```python
from build123d import *

# Parameters (mm, degrees)
CROQUIS1_W              = 50
CROQUIS1_H              = 61
SALIENTE_EXTRUIR1_DEPTH = 3
CROQUIS2_R              = 1.6
CORTAR_EXTRUIR1_DEPTH   = 40.550600501
CROQUIS4_R              = 1
CROQUIS4_W              = 23
CROQUIS4_H              = 13
CORTAR_EXTRUIR3_DEPTH   = 10
CROQUIS7_R              = 1.6
CORTAR_EXTRUIR5_DEPTH   = 10
CROQUIS5_W              = 13
CROQUIS5_H              = 7
CROQUIS5_W_2            = 26
CROQUIS5_H_2            = 11.5
CORTAR_EXTRUIR4_DEPTH   = 10
REDONDEO4_R             = 1.5
SALIENTE_EXTRUIR2_DEPTH = 3
REDONDEO3_DEPTH         = 3
REDONDEO3_2_DEPTH       = 3
REDONDEO5_R             = 2
CROQUIS9_R              = 1.6
CORTAR_EXTRUIR6_DEPTH   = 60.41214848
CORTAR_EXTRUIR7_DEPTH   = 10
MATRIZ_CRV1_OUTLINE_W   = 3.1
MATRIZ_CRV1_OUTLINE_H   = 5.1
MATRIZ_CRV1_DEPTH       = 3
CROQUIS11_W             = 5.1
CROQUIS11_H             = 3.1
CORTAR_EXTRUIR8_DEPTH   = 3


with BuildPart() as part:
    # Croquis1 → Saliente-Extruir1 (new body)
    with BuildSketch(Plane(origin=(0, 0, 0), x_dir=(1, 0, 0), z_dir=(0, 1, 0))):
        Rectangle(CROQUIS1_W, CROQUIS1_H)
    extrude(amount=SALIENTE_EXTRUIR1_DEPTH)

    # Croquis2 → Cortar-Extruir1 (cut, through all)
    with BuildSketch(Plane(origin=(0, 3, 0), x_dir=(1, 0, 0), z_dir=(0, 1, 0))):
        with Locations(Location((1, 11, 0), (0, 0, 270))):
            Circle(CROQUIS2_R)
        with Locations(Location((1, -11, 0), (0, 0, 270))):
            Circle(CROQUIS2_R)
        with BuildLine():
            Line((-16, -1.6), (-20, -1.6))
            ThreePointArc((-20, -1.6), (-21.6, 0), (-20, 1.6))
            Line((-20, 1.6), (-16, 1.6))
            ThreePointArc((-16, 1.6), (-14.4, 0), (-16, -1.6))
        make_face()
    extrude(amount=-CORTAR_EXTRUIR1_DEPTH, mode=Mode.SUBTRACT)

    # Croquis4 → Cortar-Extruir3 (cut)
    with BuildSketch(Plane(origin=(0, 3, 0), x_dir=(1, 0, 0), z_dir=(0, 1, 0))):
        with Locations(Location((-3.85, 0, 0), (0, 0, 270))):
            Circle(CROQUIS4_R)
        with Locations(Location((23.85, 0, 0), (0, 0, 270))):
            Circle(CROQUIS4_R)
        with Locations((10, 0)):
            Rectangle(CROQUIS4_W, CROQUIS4_H)
    extrude(amount=-CORTAR_EXTRUIR3_DEPTH, mode=Mode.SUBTRACT)

    # Croquis7 → Cortar-Extruir5 (cut)
    with BuildSketch(Plane(origin=(0, 3, 0), x_dir=(1, 0, 0), z_dir=(0, 1, 0))):
        with Locations(Location((5, 26, 0), (0, 0, 270))):
            Circle(CROQUIS7_R)
        with Locations(Location((5, -26, 0), (0, 0, 270))):
            Circle(CROQUIS7_R)
    extrude(amount=-CORTAR_EXTRUIR5_DEPTH, mode=Mode.SUBTRACT)

    # Croquis5 → Cortar-Extruir4 (cut)
    with BuildSketch(Plane(origin=(0, 3, 0), x_dir=(1, 0, 0), z_dir=(0, 1, 0))):
        with Locations((-11, 9.5)):
            Rectangle(CROQUIS5_W, CROQUIS5_H)
        with Locations((-11, -9.5)):
            Rectangle(CROQUIS5_W, CROQUIS5_H)
        with Locations((-12, 24.75)):
            Rectangle(CROQUIS5_W_2, CROQUIS5_H_2)
        with Locations((-12, -24.75)):
            Rectangle(CROQUIS5_W_2, CROQUIS5_H_2)
    extrude(amount=-CORTAR_EXTRUIR4_DEPTH, mode=Mode.SUBTRACT)

    # Redondeo4
    redondeo4_edges = [part.edges().sort_by_distance(p)[0] for p in [
        (-4.5, 1.5, 6),
        (-4.5, 1.5, 13),
        (-17.5, 1.5, 13),
        (-17.5, 1.5, 6),
        (-4.5, 1.5, -13),
        (-4.5, 1.5, -6),
        (-17.5, 1.5, -6),
        (-17.5, 1.5, -13),
    ]]
    fillet(redondeo4_edges, radius=REDONDEO4_R)

    # Croquis8 → Saliente-Extruir2 (add, through all)
    with BuildSketch(Plane(origin=(0, 3, 0), x_dir=(1, 0, 0), z_dir=(0, 1, 0))):
        with BuildLine():
            Line((9, -50), (19, -50))
            ThreePointArc((19, -50), (31.950013881, 0), (19, 50))
            Line((19, 50), (9, 50))
            Line((9, 50), (9, 30.5))
            Line((9, 30.5), (25, 30.5))
            Line((25, 30.5), (25, -30.5))
            Line((25, -30.5), (9, -30.5))
            Line((9, -30.5), (9, -50))
        make_face()
    extrude(amount=-SALIENTE_EXTRUIR2_DEPTH)

    # Redondeo3: read off the stored shape, not the designer's step
    # Redondeo3 outline → Redondeo3 (cut)
    with BuildSketch(Plane(origin=(0, 0, 0), x_dir=(1, 0, 0), z_dir=(0, 1, 0))):
        with BuildLine():
            ThreePointArc((5, -30.5), (2.171572875, -29.328427125), (1, -26.5))
            Line((1, -26.5), (1, -30.5))
            Line((1, -30.5), (5, -30.5))
        make_face()
        with BuildLine():
            Line((1, 30.5), (1, 26.5))
            ThreePointArc((1, 26.5), (2.171572875, 29.328427125), (5, 30.5))
            Line((5, 30.5), (1, 30.5))
        make_face()
        with BuildLine():
            Line((-25, 19), (-25, 15))
            ThreePointArc((-25, 15), (-23.828427125, 17.828427125), (-21, 19))
            Line((-21, 19), (-25, 19))
        make_face()
        with BuildLine():
            Line((-25, -19), (-21, -19))
            ThreePointArc((-21, -19), (-23.828427125, -17.828427125), (-25, -15))
            Line((-25, -15), (-25, -19))
        make_face()
    extrude(amount=REDONDEO3_DEPTH, mode=Mode.SUBTRACT)

    # Redondeo3 2 outline → Redondeo3 2 (add)
    with BuildSketch(Plane(origin=(0, 0, 0), x_dir=(1, 0, 0), z_dir=(0, 1, 0))):
        with BuildLine():
            Line((9, -30.5), (5, -30.5))
            ThreePointArc((5, -30.5), (7.828427125, -31.671572875), (9, -34.5))
            Line((9, -34.5), (9, -30.5))
        make_face()
        with BuildLine():
            ThreePointArc((9, 34.5), (7.828427125, 31.671572875), (5, 30.5))
            Line((5, 30.5), (9, 30.5))
            Line((9, 30.5), (9, 34.5))
        make_face()
        with BuildLine():
            ThreePointArc((1, 23), (-0.171572875, 20.171572875), (-3, 19))
            Line((-3, 19), (1, 19))
            Line((1, 19), (1, 23))
        make_face()
        with BuildLine():
            ThreePointArc((-3, -19), (-0.171572875, -20.171572875), (1, -23))
            Line((1, -23), (1, -19))
            Line((1, -19), (-3, -19))
        make_face()
    extrude(amount=REDONDEO3_2_DEPTH)

    # Redondeo5
    redondeo5_edges = [part.edges().sort_by_distance(p)[0] for p in [
        (9, 1.5, 50),
        (9, 1.5, -50),
        (19, 1.5, -50),
        (19, 1.5, 50),
    ]]
    fillet(redondeo5_edges, radius=REDONDEO5_R)

    # Croquis9 → Cortar-Extruir6 (cut, through all)
    with BuildSketch(Plane(origin=(0, 3, 0), x_dir=(1, 0, 0), z_dir=(0, 1, 0))):
        with Locations(Location((18.5, 18, 0), (0, 0, 270))):
            Circle(CROQUIS9_R)
        with Locations(Location((18.5, -18, 0), (0, 0, 270))):
            Circle(CROQUIS9_R)
    extrude(amount=-CORTAR_EXTRUIR6_DEPTH, mode=Mode.SUBTRACT)

    # Croquis10 → Cortar-Extruir7 (cut)
    with BuildSketch(Plane(origin=(0, 3, 0), x_dir=(1, 0, 0), z_dir=(0, 1, 0))):
        Polygon((21.502606584, 39.380484813), (23.379766719, 34.638515831), (20.497393416, 33.497496925), (18.620233281, 38.239465907), align=None)
    extrude(amount=-CORTAR_EXTRUIR7_DEPTH, mode=Mode.SUBTRACT)

    # Matriz Crv1: read off the stored shape, not the designer's step
    # Matriz Crv1 outline → Matriz Crv1 (cut)
    with BuildSketch(Plane(origin=(0, 0, 0), x_dir=(1, 0, 0), z_dir=(0, 1, 0))):
        Polygon((21.502606584, -39.380484813), (23.379766719, -34.638515831), (20.497393416, -33.497496925), (18.620233281, -38.239465907), align=None)
        Polygon((25.707954041, -27.471913222), (26.976081424, -22.532090053), (23.973443811, -21.761267526), (22.705316428, -26.701090695), align=None)
        Polygon((28.387839944, -15.130226298), (29.026941594, -10.070428962), (25.951378508, -9.68195541), (25.312276858, -14.741752746), align=None)
        with Locations((27.950013881, 0)):
            Rectangle(MATRIZ_CRV1_OUTLINE_W, MATRIZ_CRV1_OUTLINE_H)
        Polygon((29.026941594, 10.070428962), (28.387839944, 15.130226298), (25.312276858, 14.741752746), (25.951378508, 9.68195541), align=None)
        Polygon((26.976081424, 22.532090053), (25.707954041, 27.471913222), (22.705316428, 26.701090695), (23.973443811, 21.761267526), align=None)
    extrude(amount=MATRIZ_CRV1_DEPTH, mode=Mode.SUBTRACT)

    # Croquis11 → Cortar-Extruir8 (cut)
    with BuildSketch(Plane(origin=(0, 3, 0), x_dir=(1, 0, 0), z_dir=(0, 1, 0))):
        with Locations((14.885018263, 44.5)):
            Rectangle(CROQUIS11_W, CROQUIS11_H)
    cortar_extruir8 = extrude(amount=-CORTAR_EXTRUIR8_DEPTH, mode=Mode.SUBTRACT)

    # Simetría1: Cortar-Extruir8 across plane
    add(cortar_extruir8.mirror(Plane.XY), mode=Mode.SUBTRACT)


solid = part.part
```
Build history of the part. All positions in model axes, mm. A direction names the side the tool comes from. Give positions to 0.01 mm unless a question says otherwise; leave off trailing zeros. Loops run counter-clockwise (first coordinate to the right, second up) from the corner with the lowest first, then second, coordinate; pieces in that order, holes last.
1) Two-plate mould, pull along X, no slides. Class faces 1 (the face through (1, 2, 25)), 2 (the face through (9, 3, 10)), 3 (the face through (27.51, 1.48, 9.88)): released by +X, released by -X, zero draft, split by the parting line, or undercut.
Values follow:
face 1: released by -X
face 2: zero draft
face 3: undercut
2) Band-saw the part on D-D on y = 2.15. State how many separate pieces and enclosed holes the cut face has, then the cut area to 3 significant figures.
Values follow:
separate pieces: 1
enclosed holes: 21
area: 2,650 mm2
3) Band-saw the part on B-B on z = 0. List the corners of the cut face in (x, y), then the cut area to 4 significant figures.
Values follow:
outline: (-25, 0) - (-21.6, 0) - (-21.6, 3) - (-25, 3) - close; (-14.4, 0) - (-4.85, 0) - (-4.85, 3) - (-14.4, 3) - close; (-2.85, 0) - (-1.5, 0) - (-1.5, 3) - (-2.85, 3) - close; (21.5, 0) - (22.85, 0) - (22.85, 3) - (21.5, 3) - close; (24.85, 0) - (26.4, 0) - (26.4, 3) - (24.85, 3) - close; (29.5, 0) - (31.95, 0) - (31.95, 3) - (29.5, 3) - close
area: 58.95 mm2
4) Drop flat-ended pins along their axis: P1, Ø0.9, axis at x = -9.5, y = 1.5, coming from the +Z side; P2, Ø1, axis at y = 1, z = 21.5, coming from the +X side; P3, Ø0.9, axis at y = 1.5, z = 44, coming from the -X side; P4, Ø3, axis at x = 5, z = -26, coming from the +Y side. Give the stop position or say it passes through.
Values follow:
P1: stops at z = 19
P2: stops at x = 29.79
P3: stops at x = 9
P4: passes through
5) 3-axis set-ups, long thin cutter, end or side, ignore diameter. For faces 4 (the face through (9.57, 1.48, 49.4)), 5 (the face through (9, 2, -41)), 6 (the face through (20.04, 1.48, 38.8)): which of +Z, -Z, +X, -X, +Y, -Y reach the whole face in a straight line?
Values follow:
face 4: +Z, -X, +Y, -Y
face 5: -Z, -X, +Y, -Y
face 6: +Y, -Y
6) Band-saw the part on A-A on x = -9. List the corners of the cut face in (y, z), then the cut area to 3 significant figures.
Values follow:
outline: (0, -19) - (3, -19) - (3, -13) - (0, -13) - close; (0, -6) - (3, -6) - (3, 6) - (0, 6) - close; (0, 13) - (3, 13) - (3, 19) - (0, 19) - close
area: 72.0 mm2
7) Probe line 1 along X through (y, z) = (0.85, 0); line 2 along X through (y, z) = (1.85, -11); line 3 along Z through (x, y) = (21, 1.8). List the from-to ranges inside material, lowest first.
Values follow:
line 1: x = -25 to -21.6, -14.4 to -4.85, -2.85 to -1.5, 21.5 to 22.85, 24.85 to 26.4, 29.5 to 31.95
line 2: x = -25 to -17.5, -4.5 to -0.6, 2.6 to 25.78, 28.91 to 31.36
line 3: z = -46.21 to -39.18, -33.7 to -6.5, 6.5 to 33.7, 39.18 to 46.21
8) Band-saw the part on C-C on z = 18. List the corners of the cut face in (x, y) (3 decimals).
Values follow:
outline: (-23.646, 0) - (16.9, 0) - (16.9, 3) - (-23.646, 3) - close; (20.1, 0) - (30.365, 0) - (30.365, 3) - (20.1, 3) - close
